```python
from build123d import *

# Parameters (mm, degrees)
F0_W     = 203.2
F0_H     = 285.75
F0_W_2   = 190.5
F0_H_2   = 63.5
F0_W_3   = 185.42
F0_H_3   = 58.42
F1_DEPTH = 12.7
F3_W     = 6.35
F3_H     = 6.35
F3_W_2   = 44.45
F3_H_2   = 44.45
F4_DEPTH = 63.5


# Not quite as in the source:
# - the program builds the solid bodies; features that only make, move or delete a surface that nothing else refers to are left out


with BuildPart() as f1:
    # F0 (on Front) → F1 (new body)
    with BuildSketch(Plane.XZ):
        Rectangle(F0_W, F0_H)
        with Locations((0, -104.775)):
            Rectangle(F0_W_2, F0_H_2, mode=Mode.SUBTRACT)
        with Locations((0, -34.925)):
            Rectangle(F0_W_2, F0_H_2, mode=Mode.SUBTRACT)
        with Locations((0, 34.925)):
            Rectangle(F0_W_2, F0_H_2, mode=Mode.SUBTRACT)
        with Locations((0, 104.775)):
            Rectangle(F0_W_2, F0_H_2, mode=Mode.SUBTRACT)
        with Locations((0, 104.775)):
            Rectangle(F0_W_2, F0_H_2)
        with Locations((0, 104.775)):
            Rectangle(F0_W_3, F0_H_3, mode=Mode.SUBTRACT)
        with Locations((0, 34.925)):
            Rectangle(F0_W_2, F0_H_2)
        with Locations((0, 34.925)):
            Rectangle(F0_W_3, F0_H_3, mode=Mode.SUBTRACT)
        with Locations((0, -34.925)):
            Rectangle(F0_W_2, F0_H_2)
        with Locations((0, -34.925)):
            Rectangle(F0_W_3, F0_H_3, mode=Mode.SUBTRACT)
        with Locations((0, -104.775)):
            Rectangle(F0_W_2, F0_H_2)
        with Locations((0, -104.775)):
            Rectangle(F0_W_3, F0_H_3, mode=Mode.SUBTRACT)
    extrude(amount=F1_DEPTH)

    # F3 (on face) → F4 (join)
    with BuildSketch(Plane.XZ.offset(12.7)):
        with Locations((98.425, -139.7)):
            Rectangle(F3_W, F3_H)
        with Locations((73.025, -139.7)):
            Rectangle(F3_W_2, F3_H)
        with Locations((98.425, -114.3)):
            Rectangle(F3_W, F3_H_2)
        with Locations((98.425, 114.3)):
            Rectangle(F3_W, F3_H_2)
        with Locations((98.425, 139.7)):
            Rectangle(F3_W, F3_H)
        with Locations((73.025, 139.7)):
            Rectangle(F3_W_2, F3_H)
        with Locations((-98.425, -139.7)):
            Rectangle(F3_W, F3_H)
        with Locations((-73.025, -139.7)):
            Rectangle(F3_W_2, F3_H)
        with Locations((-98.425, -114.3)):
            Rectangle(F3_W, F3_H_2)
        with Locations((-98.425, 114.3)):
            Rectangle(F3_W, F3_H_2)
        with Locations((-98.425, 139.7)):
            Rectangle(F3_W, F3_H)
        with Locations((-73.025, 139.7)):
            Rectangle(F3_W_2, F3_H)
    extrude(amount=F4_DEPTH)


solid = f1.part
```
Work out the finished part from the listing and answer in its coordinate system (mm). A direction names the side the tool comes from. Give positions to 0.01 mm unless a question says otherwise; leave off trailing zeros. Write each loop counter-clockwise with the first axis right and the second up, starting at its lowest first coordinate (ties: lowest second). Pieces come first, ordered by that corner, then holes. Notation, with made-up numbers: (72.25, 54.25) -> (102.25, 54.25) arc R36 ccw to (102.25, 91.25) -> close; hole circle Ø4 at (75.25, 69.25). An arc over 180 degrees is marked (long way). Write item = value, one per line.
Q1. A tool of negligible diameter and unlimited length cuts with its end or side. For faces 3 (the flat face through (-95.25, -44, -115)), 4 (the flat face through (-50.8, -44, -140)), 5 (the flat face through (-1, -12, 142.875)), 6 (the flat face through (-1, -6, -133.985)), 7 (the flat face through (-1, -12, -142.875)), from which of +Z, -Z, +X, -X, +Y, -Y can it reach the whole face along a straight path? Write none if from no direction.
Computed values:
face_3 = -Y
face_4 = +Z, -Z, -Y
face_5 = +Z, +X, -X, +Y, -Y
face_6 = +Y, -Y
face_7 = -Z, +X, -X, +Y, -Y
Q2. Consider line 1 along X through (y, z) = (-16.5, -123.5); line 2 along Z through (x, y) = (54.5, -30) (3 decimals); line 3 along X through (y, z) = (-10.5, -112.5). Determine where each line is inside the solid, lowest interval first.
Computed values:
line_1 = -101.6 to -95.25, 95.25 to 101.6
line_2 = -142.875 to -136.525, 136.525 to 142.875
line_3 = -101.6 to -92.71, 92.71 to 101.6
Q3. Section D-D on z = -117 is taken. Determine the outline of the cut face in (x, y), and give its area (3 significant figures).
Computed values:
outline = (-101.6, -76.2) -> (-95.25, -76.2) -> (-95.25, -12.7) -> (-92.71, -12.7) -> (-92.71, 0) -> (-101.6, 0) -> close; (92.71, -12.7) -> (95.25, -12.7) -> (95.25, -76.2) -> (101.6, -76.2) -> (101.6, 0) -> (92.71, 0) -> close
area = 1,030 mm^2
Q4. For a pull along X with two mould halves and no side action, classify faces 1 (the flat face through (-8, 0, 1)), 2 (the flat face through (-73, -44, 136.525)) as pulls with the +X half, pulls with the -X half, needs draft (parallel to the pull), parting line crosses it, or undercut.
Computed values:
face_1 = needs draft
face_2 = undercut
Q5. Section A-A on y = -22 is taken. Determine the outline of the cut face in (x, z) (3 decimals).
Computed values:
outline = (-101.6, -142.875) -> (-50.8, -142.875) -> (-50.8, -136.525) -> (-95.25, -136.525) -> (-95.25, -92.075) -> (-101.6, -92.075) -> close; (-101.6, 92.075) -> (-95.25, 92.075) -> (-95.25, 136.525) -> (-50.8, 136.525) -> (-50.8, 142.875) -> (-101.6, 142.875) -> close; (50.8, -142.875) -> (101.6, -142.875) -> (101.6, -92.075) -> (95.25, -92.075) -> (95.25, -136.525) -> (50.8, -136.525) -> close; (50.8, 136.525) -> (95.25, 136.525) -> (95.25, 92.075) -> (101.6, 92.075) -> (101.6, 142.875) -> (50.8, 142.875) -> close
Q6. Section C-C on z = -40 is taken. Determine the outline of the cut face in (x, y), and give its area (3 significant figures).
Computed values:
outline = (-101.6, -12.7) -> (-92.71, -12.7) -> (-92.71, 0) -> (-101.6, 0) -> close; (92.71, -12.7) -> (101.6, -12.7) -> (101.6, 0) -> (92.71, 0) -> close
area = 226 mm^2
Q7. Section B-B on x = -70 is taken. Determine the outline of the cut face in (y, z) (3 decimals), and give its area (3 significant figures).
Computed values:
outline = (-76.2, -142.875) -> (0, -142.875) -> (0, -133.985) -> (-12.7, -133.985) -> (-12.7, -136.525) -> (-76.2, -136.525) -> close; (-76.2, 136.525) -> (-12.7, 136.525) -> (-12.7, 133.985) -> (0, 133.985) -> (0, 142.875) -> (-76.2, 142.875) -> close; (-12.7, -75.565) -> (0, -75.565) -> (0, -64.135) -> (-12.7, -64.135) -> close; (-12.7, -5.715) -> (0, -5.715) -> (0, 5.715) -> (-12.7, 5.715) -> close; (-12.7, 64.135) -> (0, 64.135) -> (0, 75.565) -> (-12.7, 75.565) -> close
area = 1,470 mm^2
